Autodesk Fusion 360 part; units mm, degrees
sketch "Sketch1" plane through (0, 0, 0) normal (0, 1, 0) x (1, 0, 0)
  circle A0 centre (0, 0) radius 16.885 construction
  circle A1 centre (0, 0) radius 17.185
  circle A2 centre (0, 0) radius 15.65
  circle A3 centre (0, 0) radius 19.385
  dimension "d1" = 33.77
  dimension "d2" = 0.3
  dimension "d3" = 31.3
  dimension "d4" = 2.5
extrude "Extrude1" add sketch "Sketch1" along normal blind 10 and the other way blind 14 contours A3
extrude "Extrude2" add sketch "Sketch1" along normal mid plane 1.5 contours A1
sketch "Sketch2" plane through (0, 0, 0) normal (0, 0, 1) x (1, 0, 0)
  line L0 (15.65, 0) -> (-15.65, 0)
  line L1 (17.185, 0) -> (-17.185, 0)
  line L2 (-15.65, 0.75) -> (15.65, 0.75)
  line L3 (-17.185, 0.75) -> (17.185, 0.75)
  line L4 (17.185, 0.75) -> (17.185, 1.75)
  arc A0 (17.185, 0.75) -> (17.185, 1.75) centre (17.185, 1.25) ccw
  line L5 (15.65, -0.75) -> (-15.65, -0.75)
  line L6 (17.185, -0.75) -> (-17.185, -0.75)
  line L7 (15.65, -0.75) -> (17.185, -4.75)
  line L8 (17.185, -0.75) -> (17.185, -4.75)
  line L9 (19.385, 10) -> (-19.385, 10)
  line L10 (17.185, 0) -> (17.185, 10) construction
  line L11 (17.185, 3.25) -> (17.185, 4.25)
  arc A1 (17.185, 3.25) -> (17.185, 4.25) centre (17.185, 3.75) ccw
  line L12 (17.185, 5.75) -> (17.185, 6.75)
  arc A2 (17.185, 5.75) -> (17.185, 6.75) centre (17.185, 6.25) ccw
  line L13 (17.185, 8.25) -> (17.185, 9.25)
  arc A3 (17.185, 8.25) -> (17.185, 9.25) centre (17.185, 8.75) ccw
  dimension "d13" = 1
  dimension "d16" = 4
  dimension "d25" = 0
  dimension "d26" = 7.5
revolve "Revolve2" cut sketch "Sketch2" angle 360 about axis through (0, 1.75, 0) along (0, 1, 0) contours L13 A3
revolve "Revolve3" add sketch "Sketch2" angle 360 about axis through (0, 1.75, 0) along (0, 1, 0) contours L6 L7 L8
revolve "Revolve4" cut sketch "Sketch2" angle 360 about axis through (0, 1.75, 0) along (0, 1, 0) contours L12 A2
revolve "Revolve5" cut sketch "Sketch2" angle 360 about axis through (0, 1.75, 0) along (0, 1, 0) contours L11 A1
revolve "Revolve6" cut sketch "Sketch2" angle 360 about axis through (0, 1.75, 0) along (0, 1, 0) contours L4 A0
fillet "Fillet1" radius 0.5 1 faces at (15.6305, 0.5, 0.7801)
ref_plane "WorkPlane1" through (0, -14, 0) normal (0, -1, 0) x (-1, 0, 0)
sketch "Sketch3" plane through (0, 10, 0) normal (0, 1, 0) x (-1, 0, 0)
  circle A0 centre (0, 0) radius 17.185
  circle A1 centre (0, 0) radius 19.385
  circle A2 centre (0, 0) radius 17.185
  circle A3 centre (0, 0) radius 19.385
  line L0 (-16.9948, 2.55) -> (16.9948, 2.55)
  line L1 (16.9948, 2.55) -> (16.9948, -2.55)
  line L2 (16.9948, -2.55) -> (-16.9948, -2.55)
  line L3 (-16.9948, -2.55) -> (-16.9948, 2.55)
  line L4 (-16.9948, 2.55) -> (16.9948, -2.55) construction
  line L5 (16.9948, 2.55) -> (-16.9948, -2.55) construction
  circle A4 centre (0, 0) radius 18.485
  line L6 (-16.9948, -2.55) -> (-18.2856, -2.7078)
  line L7 (-16.9948, 2.55) -> (-18.291, 2.6712)
  dimension "d30" = 5.1
  dimension "d31" = 1.3
extrude "Extrude3" cut sketch "Sketch3" against normal up to surface (9.25 mm away) contours A0 A2 A4 L6 L7 picked at (17.9544, 1.4876)
mirror "Mirror2" about plane through (0, -14, 0) normal (0, -1, 0) of bodies 1 merged
Verification items for the finished model (mm, model axes). A direction names the side the tool comes from. Coordinates: 2 decimals unless noted, no trailing zeros. Write each loop counter-clockwise with the first axis right and the second up, starting at its lowest first coordinate (ties: lowest second). Pieces come first, ordered by that corner, then holes. Notation, with made-up numbers: M 23.25,26.25 L 56.25,26.25 A19 cw 56.25,36.25 Z; hole C 44.25,43.25 d1. An arc over 180 degrees is marked long. One line per item, written item: value.
Item 1: Section check A-A, the plane x = 0. Record the boundary of the cut face in (y, z) (3 decimals).
Check sheet entries:
outline: M -38,-19.385 L 10,-19.385 L 10,-18.485 L 0.75,-18.485 L 0.75,-16.15 A0.5 ccw 0.25,-15.65 L -0.75,-15.65 L -4.75,-17.185 L -23.25,-17.185 L -27.25,-15.65 L -28.25,-15.65 A0.5 ccw -28.75,-16.15 L -28.75,-18.485 L -38,-18.485 Z; M -38,18.485 L -28.75,18.485 L -28.75,16.15 A0.5 ccw -28.25,15.65 L -27.25,15.65 L -23.25,17.185 L -4.75,17.185 L -0.75,15.65 L 0.25,15.65 A0.5 ccw 0.75,16.15 L 0.75,18.485 L 10,18.485 L 10,19.385 L -38,19.385 Z
Item 2: Section check C-C, the plane y = -4. Record the boundary of the cut face in (x, z) (3 decimals), plus the area to 3 significant figures.
Check sheet entries:
outline: C 0,0 d38.77; hole C 0,0 d33.794
area: 284 mm^2
Item 3: Mould release check, pull along X, two halves, no side actions. Record for faces 1 (the flat face through (16, 10, 10)), 2 (the cylindrical face through (-15.38, -14.34, -11.8)), 3 (the conical face through (7.266, -1, -13.969)): pulls with the +X half, pulls with the -X half, needs draft (parallel to the pull), parting line crosses it, or undercut.
Check sheet entries:
face 1: needs draft
face 2: parting line crosses it
face 3: undercut
Item 4: Access from +Z, -Z, +X, -X, +Y, -Y to the whole of each face (thin tool, end or side, straight path). Record for faces 4 (the flat face through (17.63, 5.44, 2.61)), 5 (the conical face through (15.02, -27, -4.73)), 6 (the cylindrical face through (17.185, -32.99, 0.036)).
Check sheet entries:
face 4: +Y
face 5: none
face 6: -Y
Item 5: Gauge pin test, flat ends, axial feed: pin 1 Ø6 at (x, y) = (15, -10.5) entering from -Z; pin 2 Ø4 at (x, y) = (3, -28) entering from -Z; pin 3 Ø12 at (y, z) = (-10, 12) entering from -X. Record the tip position at first contact, or that the pin passes through.
Check sheet entries:
pin 1: stops at z = -15.22
pin 2: stops at z = -19.36
pin 3: stops at x = -18.43
Item 6: Scan lines: line 1 along Z through (x, y) = (0, -27.9) (3 decimals); line 2 along X through (y, z) = (-11, 0) (3 decimals). Record each from-to range of solid material in increasing order.
Check sheet entries:
line 1: z = -19.385 to -15.65, 15.65 to 19.385
line 2: x = -19.385 to -17.185, 17.185 to 19.385
Item 7: Section check B-B, the plane y = -11. Record the boundary of the cut face in (x, z) (3 decimals).
Check sheet entries:
outline: C 0,0 d38.77; hole C 0,0 d34.37
